Drawing for the job (mm, zero at the part's lowest x, y, z). Round coordinates to 2 decimals unless told otherwise and drop trailing zeros. Loops run counter-clockwise (first coordinate to the right, second up) from the corner with the lowest first, then second, coordinate; pieces in that order, holes last. Notation, with made-up numbers: M 86.5,-20 L 97.5,-20 A32 cw 97.5,15 Z; hole C -21.75,22.5 d7. An arc over 180 degrees is marked long. Write each question's results on one line, items separated by ' | '.
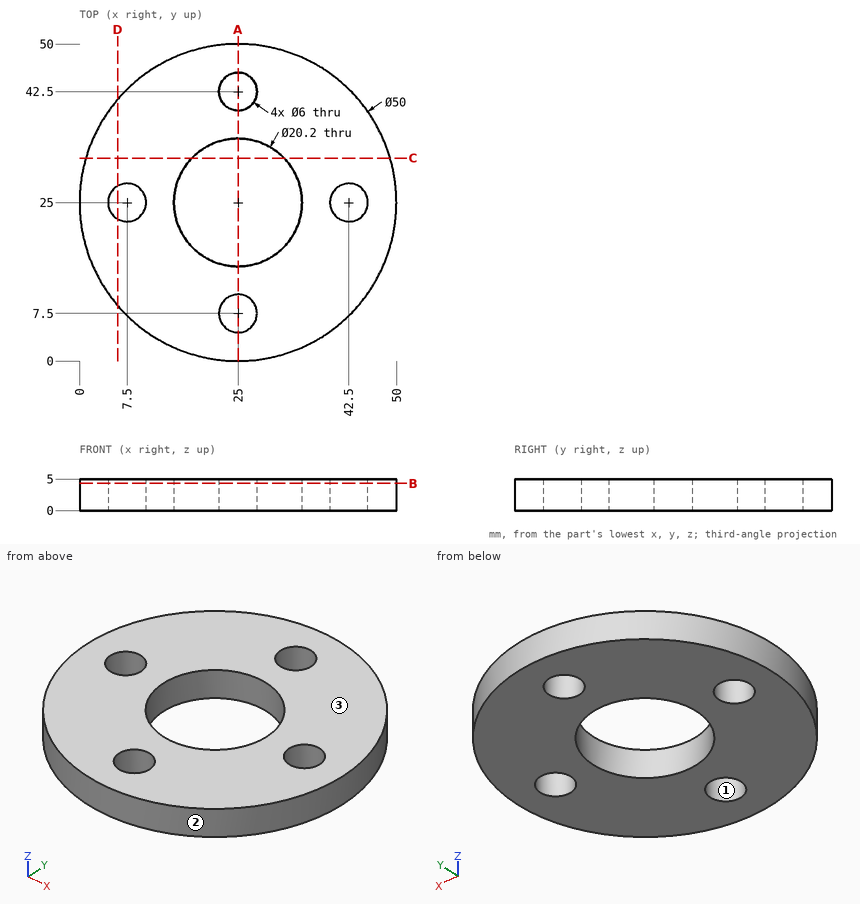
Item 1: Band-saw the part on A-A on x = 25. Give the cut face in (y, z).
Filled sheet:
outline: M 0,0 L 4.5,0 L 4.5,5 L 0,5 Z; M 10.5,0 L 14.9,0 L 14.9,5 L 10.5,5 Z; M 35.1,0 L 39.5,0 L 39.5,5 L 35.1,5 Z; M 45.5,0 L 50,0 L 50,5 L 45.5,5 Z
Item 2: Wall check: L1, parallel to Y at x = 25, z = 3.95; L2, parallel to X at y = 24, z = 1.1; L3, parallel to Y at x = 23, z = 2.6. Give the ranges that are in metal, low to high.
Filled sheet:
L1: 0 to 4.5, 10.5 to 14.9, 35.1 to 39.5, 45.5 to 50 | L2: 0.02 to 4.67, 10.33 to 14.95, 35.05 to 39.67, 45.33 to 49.98 | L3: 0.08 to 5.26, 9.74 to 15.1, 34.9 to 40.26, 44.74 to 49.92
Item 3: Band-saw the part on C-C on y = 32. Give the cut face in (x, z).
Filled sheet:
outline: M 1,0 L 17.72,0 L 17.72,5 L 1,5 Z; M 32.28,0 L 49,0 L 49,5 L 32.28,5 Z
Item 4: Band-saw the part on B-B on z = 4.3. Give the cut face in (x, y).
Filled sheet:
outline: C 25,25 d50; hole C 7.5,25 d6; hole C 25,25 d20.2; hole C 25,7.5 d6; hole C 25,42.5 d6; hole C 42.5,25 d6
Item 5: Band-saw the part on D-D on x = 6. Give the cut face in (y, z).
Filled sheet:
outline: M 8.75,0 L 22.4,0 L 22.4,5 L 8.75,5 Z; M 27.6,0 L 41.25,0 L 41.25,5 L 27.6,5 Z
Item 6: Two-plate mould, pull along Y, no slides. Class the marked faces 1, 2 and 3: +Y half, -Y half, draft (parallel to the pull), parting line (faces both ways), or undercut.
Filled sheet:
face 1: undercut | face 2: parting line | face 3: draft
Item 7: Drop flat-ended pins along their axis: P1, Ø1, axis at x = 41.5, z = 4, coming from the -Y side; P2, Ø1.5, axis at y = 20.5, z = 0.5, coming from the +X side; P3, Ø1, axis at y = 18, z = 2.5, coming from the -X side. Give the stop position or say it passes through.
Filled sheet:
P1: y = 5.79 | P2: x = 49.72 | P3: x = 0.86
